Read the model definition and answer for the solid it produces. Units are mm, in the model's axes. Face numbers are marked on the shaded views. Give positions to 0.01 mm unless a question says otherwise; leave off trailing zeros. Loops run counter-clockwise (first coordinate to the right, second up) from the corner with the lowest first, then second, coordinate; pieces in that order, holes last. Notation, with made-up numbers: (9, -10.75) - (38, -10.75) arc R17 ccw to (38, 3.25) - close; hole circle Ø8 at (68, 54.5). An arc over 180 degrees is marked (long way). Put each result on its own line as item: value. Start each with the question number.
1. Consider L1, parallel to X at y = 12, z = -2.5; L2, parallel to Y at x = -67, z = -1.5; L3, parallel to Z at x = -70, y = 18.5. Determine where each line is inside the solid, lowest interval first. Write a range as from..to.
2. A cutting plane is placed at D-D, the plane y = 10. Determine the outline of the cut face in (x, z), plus the area to 3 significant figures.
3. A cutting plane is placed at C-C, the plane y = 30. Determine the outline of the cut face in (x, z).
4. A cutting plane is placed at A-A, the plane z = -0.75. Determine the outline of the cut face in (x, y), plus the area to 3 significant figures.
5. For a pull along Y with two mould halves and no side action, classify the marked faces 1, 2 and 3 as released by +Y, released by -Y, zero draft, split by the parting line, or undercut.
6. A cutting plane is placed at B-B, the plane x = -64.5. Determine the outline of the cut face in (y, z).
7. Given pin 1 Ø2 at (y, z) = (10, 0.5) entering from +X; pin 2 Ø0.9 at (x, z) = (-40, 1) entering from +Y; pin 3 Ø0.5 at (x, z) = (-65.5, 1.5) entering from -Y; pin 4 Ø4 at (x, y) = (-66.06, 10) entering from -Z, each flat-ended and moving along its own axis, determine where each tip first touches the part or whether it passes through.
```python
from build123d import *

# Parameters (mm, degrees)
F0_W     = 6
F0_H     = 8
F0_H_2   = 5.5
F0_H_3   = 7.5
F0_W_2   = 7
F0_H_4   = 6
F0_W_3   = 7.5
F0_W_4   = 5.5
F0_W_5   = 8
F0_H_5   = 7
F1_DEPTH = 4.5
F2_DEPTH = 1.8
F3_D     = 5.2
F4_R     = 5


with BuildPart() as f1:
    # F0 (on Top) → F1 (new body)
    with BuildSketch(Plane.XY):
        Polygon((-69.0596391448, 47.1421356237), (-76.0596391448, 54.1421356237), (-76.0596391448, 13), (-69.0596391448, 13), (-69.0596391448, 20.5), (-69.0596391448, 26), (-69.0596391448, 34), align=None)
        Polygon((-63.0596391448, 41.1421356237), (-69.0596391448, 47.1421356237), (-69.0596391448, 34), (-63.0596391448, 34), align=None)
        with Locations((-66.0596391448, 30)):
            Rectangle(F0_W, F0_H)
        with Locations((-66.0596391448, 23.25)):
            Rectangle(F0_W, F0_H_2)
        with Locations((-66.0596391448, 16.75)):
            Rectangle(F0_W, F0_H_3)
        Polygon((-34.9175035211, 13), (-63.0596391448, 41.1421356237), (-63.0596391448, 34), (-63.0596391448, 26), (-63.0596391448, 20.5), (-63.0596391448, 13), (-55.5596391448, 13), (-50.0596391448, 13), (-42.0596391448, 13), align=None)
        with Locations((-72.5596391448, 10)):
            Rectangle(F0_W_2, F0_H_4)
        with Locations((-66.0596391448, 10)):
            Rectangle(F0_W, F0_H_4)
        with Locations((-59.3096391448, 10)):
            Rectangle(F0_W_3, F0_H_4)
        with Locations((-52.8096391448, 10)):
            Rectangle(F0_W_4, F0_H_4)
        with Locations((-46.0596391448, 10)):
            Rectangle(F0_W_5, F0_H_4)
        Polygon((-28.9175035211, 7), (-34.9175035211, 13), (-42.0596391448, 13), (-42.0596391448, 7), align=None)
        Polygon((-55.5596391448, 7), (-63.0596391448, 7), (-63.0596391448, 0), (-21.9175035211, 0), (-28.9175035211, 7), (-42.0596391448, 7), (-50.0596391448, 7), align=None)
        with Locations((-66.0596391448, 3.5)):
            Rectangle(F0_W, F0_H_5)
        with Locations((-72.5596391448, 3.5)):
            Rectangle(F0_W_2, F0_H_5)
    extrude(amount=-F1_DEPTH)

    # F0 (on Top) → F2 (join)
    with BuildSketch(Plane.XY):
        Polygon((-63.0596391448, 41.1421356237), (-69.0596391448, 47.1421356237), (-69.0596391448, 34), (-63.0596391448, 34), align=None)
        with Locations((-66.0596391448, 23.25)):
            Rectangle(F0_W, F0_H_2)
        with Locations((-52.8096391448, 10)):
            Rectangle(F0_W_4, F0_H_4)
        Polygon((-28.9175035211, 7), (-34.9175035211, 13), (-42.0596391448, 13), (-42.0596391448, 7), align=None)
    extrude(amount=F2_DEPTH)

    # F3 (through all)
    with Locations(Plane.XY):
        with Locations((-66.0596391448, 30), (-66.0596391448, 10), (-46.0596391448, 10)):
            Hole(F3_D / 2)

    # F4
    f4_edges = [f1.edges().sort_by_distance(p)[0] for p in [
        (-21.917504, 0, -2.25),
        (-76.059639, 0, -2.25),
        (-76.059639, 54.142136, -2.25),
    ]]
    fillet(f4_edges, radius=F4_R)


solid = f1.part
```
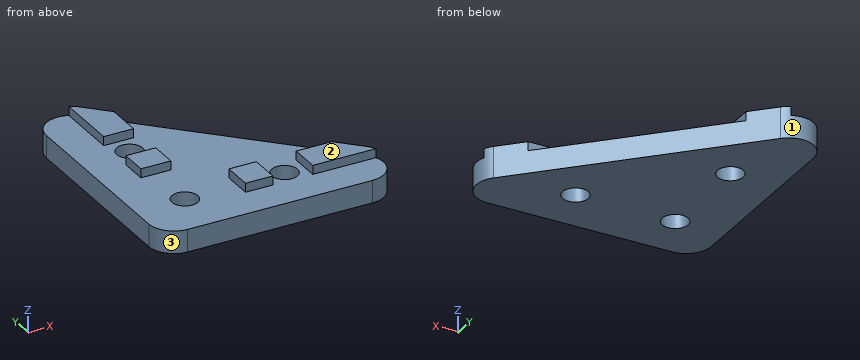
Return value:
1. L1: x = -76.06..-67.72, -64.4..-47.72, -44.4..-33.92
1. L2: y = 0..7.58, 12.42..27.58, 32.42..45.08
1. L3: z = -4.5..0
2. outline: (-76.06, -4.5) - (-68.66, -4.5) - (-68.66, 0) - (-76.06, 0) - close; (-63.46, -4.5) - (-48.66, -4.5) - (-48.66, 0) - (-50.06, 0) - (-50.06, 1.8) - (-55.56, 1.8) - (-55.56, 0) - (-63.46, 0) - close; (-43.46, -4.5) - (-31.92, -4.5) - (-31.92, 1.8) - (-42.06, 1.8) - (-42.06, 0) - (-43.46, 0) - close
2. area: 180 mm2
3. outline: (-76.06, -4.5) - (-68.66, -4.5) - (-68.66, 0) - (-76.06, 0) - close; (-63.46, -4.5) - (-51.92, -4.5) - (-51.92, 0) - (-63.46, 0) - close
4. outline: (-76.06, 5) arc R5 ccw to (-71.06, 0) - (-33.99, 0) arc R5 ccw to (-30.45, 8.54) - (-67.52, 45.61) arc R5 ccw to (-76.06, 42.07) - close; hole circle Ø5.2 at (-66.06, 10); hole circle Ø5.2 at (-66.06, 30); hole circle Ø5.2 at (-46.06, 10)
4. area: 1,330 mm2
5. face 1: released by +Y
5. face 2: zero draft
5. face 3: released by -Y
6. outline: (0, -4.5) - (7.92, -4.5) - (7.92, 0) - (0, 0) - close; (12.08, -4.5) - (27.92, -4.5) - (27.92, 0) - (26, 0) - (26, 1.8) - (20.5, 1.8) - (20.5, 0) - (12.08, 0) - close; (32.08, -4.5) - (42.58, -4.5) - (42.58, 1.8) - (34, 1.8) - (34, 0) - (32.08, 0) - close
7. pin 1: stops at x = -30.92
7. pin 2: stops at y = 13
7. pin 3: stops at y = 20.5
7. pin 4: passes through
